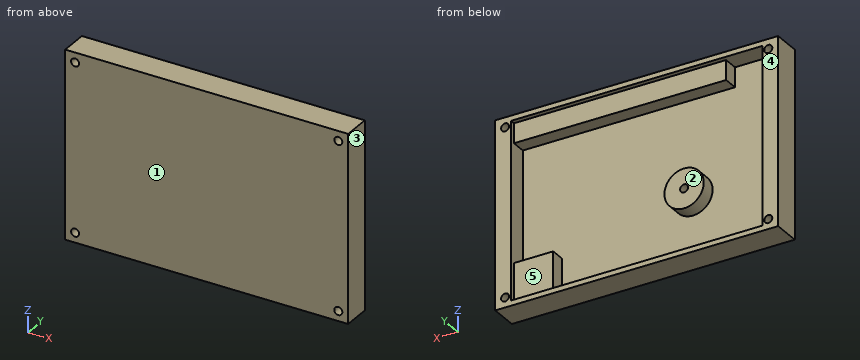
```python
from build123d import *

# Parameters (mm, degrees)
SKETCH1_W           = 91.44
SKETCH1_H           = 60.452
BOSS_EXTRUDE1_DEPTH = 8.89
SKETCH2_W           = 81.28
SKETCH2_H           = 57.15
CUT_EXTRUDE1_DEPTH  = 1.6002
SKETCH3_R           = 6.35
SKETCH3_R_2         = 1.28905
CUT_EXTRUDE2_DEPTH  = 4.7498
SKETCH4_R           = 1.28905
CUT_EXTRUDE3_DEPTH  = 56.524423239


with BuildPart() as part:
    # Sketch1 → Boss-Extrude1 (new body)
    with BuildSketch(Plane(origin=(0, 0, 0), x_dir=(1, 0, 0), z_dir=(0, 1, 0))):
        Rectangle(SKETCH1_W, SKETCH1_H)
    extrude(amount=BOSS_EXTRUDE1_DEPTH)

    # Sketch2 → Cut-Extrude1 (cut)
    with BuildSketch(Plane(origin=(0, 8.89, 0), x_dir=(1, 0, 0), z_dir=(0, 1, 0))):
        Rectangle(SKETCH2_W, SKETCH2_H)
    extrude(amount=-CUT_EXTRUDE1_DEPTH, mode=Mode.SUBTRACT)

    # Sketch3 → Cut-Extrude2 (cut)
    with BuildSketch(Plane(origin=(0, 7.2898, 0), x_dir=(1, 0, 0), z_dir=(0, 1, 0))):
        Polygon((-40.64, 28.575), (27.94, 28.575), (27.94, 15.875), (40.64, 15.875), (40.64, -22.225), (-27.94, -22.225), (-27.94, -28.575), (-40.64, -28.575), (-40.64, -22.225), align=None)
        with Locations(Location((-14.351, 8.255, 0), (0, 0, 270))):
            Circle(SKETCH3_R, mode=Mode.SUBTRACT)
        with Locations(Location((-14.351, 8.255, 0), (0, 0, 270))):
            Circle(SKETCH3_R_2)
    extrude(amount=-CUT_EXTRUDE2_DEPTH, mode=Mode.SUBTRACT)

    # Sketch4 → Cut-Extrude3 (cut, through all)
    with BuildSketch(Plane(origin=(0, 8.89, 0), x_dir=(1, 0, 0), z_dir=(0, 1, 0))):
        with Locations(Location((-42.545, 27.051, 0), (0, 0, 270))):
            Circle(SKETCH4_R)
        with Locations(Location((-42.545, -27.051, 0), (0, 0, 270))):
            Circle(SKETCH4_R)
        with Locations(Location((42.545, -27.051, 0), (0, 0, 270))):
            Circle(SKETCH4_R)
        with Locations(Location((42.545, 27.051, 0), (0, 0, 270))):
            Circle(SKETCH4_R)
    extrude(amount=-CUT_EXTRUDE3_DEPTH, mode=Mode.SUBTRACT)


solid = part.part
```
Could you check a few things on this model? Use its own coordinates, in mm. Face numbers are marked on the shaded views. A direction names the side the tool comes from. Round coordinates to 2 decimals unless told otherwise and drop trailing zeros. Loops run counter-clockwise (first coordinate to the right, second up) from the corner with the lowest first, then second, coordinate; pieces in that order, holes last. Notation, with made-up numbers: M -17,84.5 L 4,84.5 A29 ccw 4,109.5 Z; hole C -25,-39 d8. An arc over 180 degrees is marked long. Put each result on its own line as item: value.
Q1. Imagine slicing it at B-B (z = 18). Write out the boundary of the cut face in (x, y), then the cut area to 3 significant figures.
Check result:
outline: M -45.72,0 L 45.72,0 L 45.72,8.89 L 40.64,8.89 L 40.64,2.54 L -40.64,2.54 L -40.64,8.89 L -45.72,8.89 Z
area: 297 mm2
Q2. Imagine slicing it at C-C (x = 4.5). Write out the boundary of the cut face in (y, z) (3 decimals), then the cut area to 3 significant figures.
Check result:
outline: M 0,-30.226 L 8.89,-30.226 L 8.89,-28.575 L 2.54,-28.575 L 2.54,22.225 L 7.29,22.225 L 7.29,28.575 L 8.89,28.575 L 8.89,30.226 L 0,30.226 Z
area: 205 mm2
Q3. Thinking about a two-plate mould opening in X: for the marked faces 3, 4 and 5, which applies, released by +X, released by -X, zero draft, split by the parting line, or undercut?
Check result:
face 3: released by +X
face 4: zero draft
face 5: undercut
Q4. Imagine slicing it at D-D (z = -11). Write out the boundary of the cut face in (x, y), then the cut area to 3 significant figures.
Check result:
outline: M -45.72,0 L 45.72,0 L 45.72,8.89 L 40.64,8.89 L 40.64,2.54 L -8.62,2.54 L -8.62,7.29 L -20.08,7.29 L -20.08,2.54 L -40.64,2.54 L -40.64,8.89 L -45.72,8.89 Z
area: 351 mm2
Q5. Imagine slicing it at A-A (y = 4.5). Write out the boundary of the cut face in (x, z) (3 decimals), then the cut area to 3 significant figures.
Check result:
outline: M -45.72,-30.226 L 45.72,-30.226 L 45.72,30.226 L -45.72,30.226 Z; C -14.351,-8.255 d12.7; hole C -42.545,-27.051 d2.578; hole C -42.545,27.051 d2.578; hole M -40.64,-28.575 L 27.94,-28.575 L 27.94,-15.875 L 40.64,-15.875 L 40.64,22.225 L -27.94,22.225 L -27.94,28.575 L -40.64,28.575 Z; hole C -14.351,-8.255 d2.578; hole C 42.545,-27.051 d2.578; hole C 42.545,27.051 d2.578
area: 1,580 mm2
Q6. I need wall thicknesses on probe 1 along Z at (x, y) = (39, 4) (3 decimals); probe 2 along Z at (x, y) = (8, 5.75) (3 decimals); probe 3 along X at (y, z) = (4.5, -9). Which ranges of each line are inside material? Lowest first, please.
Check result:
probe 1: -30.226 to -15.875, 22.225 to 30.226
probe 2: -30.226 to -28.575, 22.225 to 30.226
probe 3: -45.72 to -40.64, -20.66 to -15.4, -13.3 to -8.04, 40.64 to 45.72
Q7. For pin 1 (10 mm diameter, centred on x = -17.5, z = -6.5, fed in from +Y); pin 2 (17 mm diameter, centred on x = 13.5, z = 13.5, fed in from +Y), each with a flat end and sliding along its axis, tell me the tip position at first contact or that it passes through.
Check result:
pin 1: y = 7.29
pin 2: y = 2.54
Q8. On a 3-axis mill with a long thin cutter (end or side, diameter ignored), from which of +Z, -Z, +X, -X, +Y, -Y can I reach the whole of each face in a straight line? I mean the marked faces 1 and 2. Say none if no direction works.
Check result:
face 1: +Z, -Z, +X, -X, -Y
face 2: +Y
